Autodesk Inventor part; units mm, degrees
ref_plane "YZ Plane" through (0, 0, 0) normal (1, 0, 0) x (0, 1, 0)
ref_plane "XZ Plane" through (0, 0, 0) normal (0, 1, 0) x (-1, 0, 0)
ref_plane "XY Plane" through (0, 0, 0) normal (0, 0, 1) x (1, 0, 0)
sketch "スケッチ1" plane through (0, 0, 0) normal (0, 1, 0) x (-1, 0, 0)
  line L0 (0, 0) -> (40, 0)
  line L1 (40, 0) -> (40, -26.8558)
  line L2 (40, -26.8558) -> (0, -26.8558)
  line L3 (0, -26.8558) -> (0, 0)
  circle A0 centre (20, -26.8558) radius 15
  line L4 (20, -26.8558) -> (20, 0)
  line L5 (40, -23.6058) -> (40, -26.8558)
  line L6 (0, -23.6058) -> (0, -26.8558)
  circle A1 centre (20, -26.8558) radius 17
  line L7 (40, -26.8558) -> (46, -26.8558)
  line L8 (46, -26.8558) -> (46, -23.6058)
  line L9 (46, -23.6058) -> (40, -23.6058)
  line L10 (40, -23.6058) -> (40, -26.8558)
  line L11 (0, -23.6058) -> (0, -26.8558)
  line L12 (0, -26.8558) -> (-6, -26.8558)
  line L13 (-6, -26.8558) -> (-6, -23.6058)
  line L14 (-6, -23.6058) -> (0, -23.6058)
  line L15 (0, -23.6058) -> (0, -26.8558)
  point P0 (35, -26.8558)
  point P1 (5, -26.8558)
  dimension "d0" = 40
  dimension "d1" = 30
  dimension "d16" = 34
  dimension "d18" = 6
  dimension "d19" = 3.25
extrude "押し出し1" add sketch "スケッチ1" along normal blind 1 contours L0 L4 A1 L2 L3 | L0 L1 L2 A1 L4 | A1 L2 A0 L4 | L4 A0 L2 A1 | L4 L2 A0 | A0 L2 L4
fillet "フィレット1" radius 15 2 edges at (-40, 0.5, 0) (0, 0.5, 0)
extrude "押し出し4" add sketch "スケッチ1" along normal blind 9 contours L3 L12 L13 L14 | L9 L8 L7 L1
sketch "スケッチ7" plane through (6, 0, -26.8558) normal (0, 0, -1) x (-1, 0, 0)
  circle A0 centre (3, 6) radius 1.375
  line L0 (6, 1) -> (6, 9)
  line L1 (0, 9) -> (6, 9)
  circle A1 centre (49.4019, 6) radius 1.375
  line L2 (46, 9) -> (52, 9)
  line L3 (52, 0) -> (52, 9)
  point P0 (6, 0)
  point P1 (3, 9)
  point P2 (52, 4.5)
  dimension "d22" = 2.75
  dimension "d23" = 3
  dimension "d24" = 3
  dimension "d25" = 2.75
  dimension "d26" = 3
  dimension "d27" = 3
extrude "押し出し5" cut sketch "スケッチ7" against normal blind 6
extrude "押し出し6" cut sketch "スケッチ1" along normal blind 1 contours L4 L2 A0 | A0 L2 L4
sketch "スケッチ9" plane through (6, 9, -26.8558) normal (0, 0, -1) x (-1, 0, 0)
  line L0 (6, -8) -> (6, 0)
  line L1 (6, -8) -> (11, -8)
  line L2 (11, -8) -> (11, -7)
  line L3 (11, -7) -> (6, -7)
  line L4 (6, -7) -> (6, -8)
  line L5 (6, 0) -> (11, -7)
  line L6 (41, -8) -> (41, -9)
  line L7 (52, 0) -> (46, 0)
  line L8 (46, -8) -> (46, 0)
  line L9 (46, -8) -> (41, -8)
  line L10 (41, -8) -> (41, -7)
  line L11 (41, -7) -> (46, -7)
  line L12 (46, -7) -> (46, -8)
  line L13 (46, 0) -> (41, -7)
  point P0 (6, -9)
  dimension "d32" = 5
  dimension "d33" = 1
  dimension "d38" = 5
extrude "押し出し7" add sketch "スケッチ9" against normal blind 3.25
properties part number "PartsForRaspibase"
Verification items for the finished model (mm, model axes). A direction names the side the tool comes from. Coordinates: 2 decimals unless noted, no trailing zeros. Order: outer loops, then holes, each group sorted by start corner. A loop starts at its lowest first (then second) coordinate and runs counter-clockwise, first axis right, second up. Notation, with made-up numbers: (37.5, 4) -> (50.5, 4) arc R16 ccw to (50.5, 32) -> close; hole circle Ø5 at (30, 53.5). An arc over 180 degrees is marked (long way). Answer as CSV lines item,"result". Start each with the question number.
1) Gauge pin test, flat ends, axial feed: pin 1 Ø1 at (x, y) = (-36.5, 8) entering from +Z; pin 2 Ø1.1 at (y, z) = (0.5, -19.5) entering from +X; pin 3 Ø0.5 at (y, z) = (0.5, -17) entering from -X; pin 4 Ø8 at (x, z) = (-39, -20.5) entering from +Y. Record the tip position at first contact, or that the pin passes through.
2) Cross-section at A-A, the plane x = 3. Record the boundary of the cut face in (y, z) (3 decimals), then the cut area to 3 significant figures.
3) Cross-section at D-D, the plane x = -20. Record the boundary of the cut face in (y, z), then the cut area to 3 significant figures.
4) Cross-section at C-C, the plane y = 6. Record the boundary of the cut face in (x, z) (3 decimals).
5) Material ranges on L1, parallel to Y at x = 3, z = -25.3 (3 decimals); L2, parallel to Z at x = -41.5, y = 3.75; L3, parallel to Y at x = -36.5, z = -11, recorded low to high. Write a range as [from, to].
6) Release check for a two-part mould opening along X. For faces 4 (the face through (-37.5, 5.5, -25.3)), 5 (the face through (-4.51, 0.51, -4.28)), 6 (the face through (-42, 5, -23.606)) record: released by +X, released by -X, zero draft, split by the parting line, or undercut.
7) Cross-section at B-B, the plane z = -19. Record the boundary of the cut face in (x, y).
8) Set-up check for faces 1 (the face through (-40, 0.5, -19.2)), 2 (the face through (-5, 1.5, -25.3)), 3 (the face through (0, 0.5, -19.4)): record each of +Z, -Z, +X, -X, +Y, -Y from which the full face is reachable in a straight line by a thin tool's end or side.
Conclusion:
1,pin 1,"passes through"
1,pin 2,"stops at x = 0"
1,pin 3,"stops at x = -40"
1,pin 4,"stops at y = 9"
2,outline,"(0, -26.856) -> (4.625, -26.856) -> (4.625, -23.606) -> (0, -23.606) -> close; (7.375, -26.856) -> (9, -26.856) -> (9, -23.606) -> (7.375, -23.606) -> close"
2,area,"20.3 mm²"
3,outline,"(0, -11.86) -> (1, -11.86) -> (1, 0) -> (0, 0) -> close"
3,area,"11.9 mm²"
4,outline,"(-46, -26.856) -> (-44.777, -26.856) -> (-44.777, -23.606) -> (-46, -23.606) -> close; (-42.027, -26.856) -> (-37.857, -26.856) -> (-37.857, -23.606) -> (-42.027, -23.606) -> close; (-2.143, -26.856) -> (1.625, -26.856) -> (1.625, -23.606) -> (-2.143, -23.606) -> close; (4.375, -26.856) -> (6, -26.856) -> (6, -23.606) -> (4.375, -23.606) -> close"
5,L1,"y = [0, 4.625], [7.375, 9]"
5,L2,"z = [-26.86, -23.61]"
5,L3,"y = [0, 1]"
6,face 4,"undercut"
6,face 5,"released by +X"
6,face 6,"zero draft"
7,outline,"(-40, 0) -> (-32.78, 0) -> (-32.78, 1) -> (-40, 1) -> close; (-7.22, 0) -> (0, 0) -> (0, 1) -> (-7.22, 1) -> close"
8,face 1,"+Z, -X, +Y, -Y"
8,face 2,"+Z, -Z, +Y"
8,face 3,"+Z, +X, +Y, -Y"
